The model under review builds one solid part; all positions refer to its coordinate system, in mm. A direction names the side the tool comes from. Give positions to 0.01 mm unless a question says otherwise; leave off trailing zeros. Write each loop counter-clockwise with the first axis right and the second up, starting at its lowest first coordinate (ties: lowest second). Pieces come first, ordered by that corner, then holes. Notation, with made-up numbers: (10, -36.5) -> (68, -36.5) arc R21 cw to (68, -4.5) -> close; hole circle Ø8 at (-19, -4). An arc over 180 degrees is marked (long way). Use CSV: the item, a comma, the result in double quotes.
```python
from build123d import *

# Parameters (mm, degrees)
F2_R     = 12.7
F3_DEPTH = 80.0862


with BuildPart() as f1:
    # F0 (on Right) → F1 (revolve)
    with BuildSketch(Plane.YZ):
        with BuildLine():
            Line((0, 40.005), (-25.273, 40.005))
            Line((-25.273, 40.005), (-25.273, 9.361256))
            Line((-25.273, 9.361256), (-25.430815, 9.203441))
            ThreePointArc((-25.430815, 9.203441), (-25.654, 8.664625), (-25.430815, 8.12581))
            Line((-25.430815, 8.12581), (-17.52819, 0.223185))
            ThreePointArc((-17.52819, 0.223185), (-16.989375, 0), (-16.450559, 0.223185))
            Line((-16.450559, 0.223185), (-8.009118, 8.664625))
            Line((-8.009118, 8.664625), (0, 8.664625))
            Line((0, 8.664625), (0, 40.005))
        make_face()
    revolve(axis=Axis((0, 0, 24.334813), (0, 0, -1)))

    # F2 (on face) → F3 (join)
    with BuildSketch(Plane.XY.offset(40.005)):
        Circle(F2_R)
    extrude(amount=F3_DEPTH)


solid = f1.part
```
Q1. Consider section C-C (z = 82). Write out the cut boundary in (x, y), then the cut area to 3 significant figures.
Derived:
outline,"circle Ø25.4 at (0, 0)"
area,"507 mm2"
Q2. To check wall thickness, follow probe 1 along Y at (x, z) = (-1, 29); probe 2 along Z at (x, y) = (20.5, -15). State the ranges of each line that lie inside material, in increasing order.
Derived:
probe 1,"y = -25.25 to 25.25"
probe 2,"z = 8.1 to 9.23"
Q3. The part is to be moulded in two halves that separate along Y. For faces 3 (the flat face through (0, 0, 8.665)), 4 (the cylindrical face through (-2.75, -12.4, 79.49)), 5 (the flat face through (0, 0, 120.091)), say which applies: pulls with the +Y half, pulls with the -Y half, needs draft (parallel to the pull), parting line crosses it, or undercut.
Derived:
face 3,"undercut"
face 4,"parting line crosses it"
face 5,"needs draft"
Q4. Consider section A-A (x = 0). Write out the cut boundary in (y, z) (3 decimals), then the cut area to 3 significant figures.
Derived:
outline,"(-25.431, 8.126) -> (-17.528, 0.223) arc R0.762 ccw to (-16.451, 0.223) -> (-8.009, 8.665) -> (8.009, 8.665) -> (16.451, 0.223) arc R0.762 ccw to (17.528, 0.223) -> (25.431, 8.126) arc R0.762 ccw to (25.431, 9.203) -> (25.273, 9.361) -> (25.273, 40.005) -> (12.7, 40.005) -> (12.7, 120.091) -> (-12.7, 120.091) -> (-12.7, 40.005) -> (-25.273, 40.005) -> (-25.273, 9.361) -> (-25.431, 9.203) arc R0.762 ccw to start"
area,"3,780 mm2"
Q5. Consider section D-D (z = 35). Write out the cut boundary in (x, y), then the cut area to 3 significant figures.
Derived:
outline,"circle Ø50.55 at (0, 0)"
area,"2,010 mm2"
Q6. Machinability: for faces 1 (the cylindrical face through (22.4, -11.7, 24.5)), 2 (the conical face through (6.86, -16.55, 0.61)), which of the approach directions +Z, -Z, +X, -X, +Y, -Y give a long, thin tool a straight path to every point of the face, cutting with its end or side? Answer none if there is none.
Derived:
face 1,"+Z"
face 2,"-Z"
Q7. Insertion check: pin 1 (17.5 mm diameter, centred on x = 1.5, y = -1, fed in from -Z); pin 2 (6 mm diameter, centred on x = 17, z = 46.5, fed in from -Y); pin 3 (4 mm diameter, centred on y = 12, z = 83, fed in from -X); pin 4 (3 mm diameter, centred on y = -9, z = 99.5, fed in from +X). Each pin has a flat end and moves straight along its axis. Give the tip position at first contact, or say it passes through.
Derived:
pin 1,"stops at z = 6.12"
pin 2,"passes through"
pin 3,"stops at x = -7.83"
pin 4,"stops at x = 10.25"
